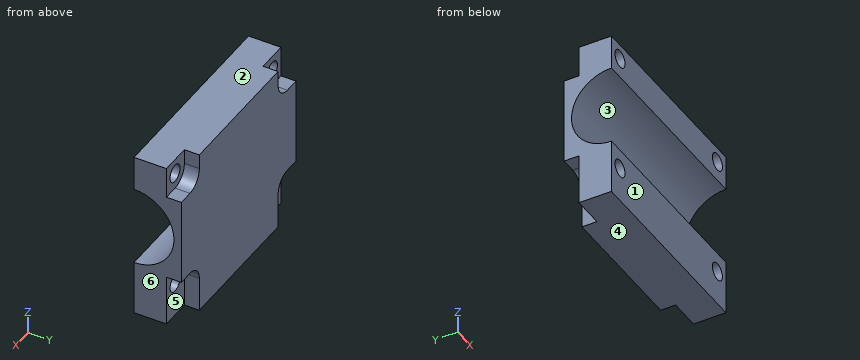
from build123d import *

# Parameters (mm, degrees)
SKETCH1_W            = 40
SKETCH1_H            = 34
SKETCH1_R            = 1.75
BOSS_EXTRUDE1_DEPTH  = 9.5
SKETCH2_R            = 8
CUT_EXTRUDE1_DEPTH   = 46.290727528
CUT_EXTRUDE2_DEPTH   = 3
MIRROR2_COPY_1_DEPTH = 3
SKETCH4_W            = 6.25
SKETCH4_H            = 4
CUT_EXTRUDE3_DEPTH   = 3


with BuildPart() as part:
    # Sketch1 → Boss-Extrude1 (new body)
    with BuildSketch(Plane(origin=(0, 0, 0), x_dir=(1, 0, 0), z_dir=(0, 1, 0))):
        with Locations((0, 2)):
            Rectangle(SKETCH1_W, SKETCH1_H)
        with Locations(Location((-17, 12, 0), (0, 0, 270))):
            Circle(SKETCH1_R, mode=Mode.SUBTRACT)
        with Locations(Location((17, 12, 0), (0, 0, 270))):
            Circle(SKETCH1_R, mode=Mode.SUBTRACT)
        with Locations(Location((17, -12, 0), (0, 0, 270))):
            Circle(SKETCH1_R, mode=Mode.SUBTRACT)
        with Locations(Location((-17, -12, 0), (0, 0, 270))):
            Circle(SKETCH1_R, mode=Mode.SUBTRACT)
    extrude(amount=BOSS_EXTRUDE1_DEPTH)

    # Sketch2 → Cut-Extrude1 (cut, through all)
    with BuildSketch(Plane(origin=(20, 0, 0), x_dir=(0, 0, -1), z_dir=(1, 0, 0))):
        Circle(SKETCH2_R)
    extrude(amount=-CUT_EXTRUDE1_DEPTH, mode=Mode.SUBTRACT)

    # Sketch3 → Cut-Extrude2 (cut)
    with BuildSketch(Plane(origin=(0, 9.5, 0), x_dir=(1, 0, 0), z_dir=(0, 1, 0))):
        with BuildLine():
            Line((-17, -8.75), (-20, -8.75))
            Line((-20, -8.75), (-20, -15))
            Line((-20, -15), (-13.75, -15))
            Line((-13.75, -15), (-13.75, -12))
            ThreePointArc((-13.75, -12), (-14.701902961, -9.701902961), (-17, -8.75))
        make_face()
    cut_extrude2 = extrude(amount=-CUT_EXTRUDE2_DEPTH, mode=Mode.SUBTRACT)

    # Mirror1: Cut-Extrude2 across plane
    add(cut_extrude2.mirror(Plane(origin=(0, 0, 0), x_dir=(0, 0, 1), z_dir=(1, 0, 0))), mode=Mode.SUBTRACT)

    # Mirror2: Cut-Extrude2 across plane
    add(cut_extrude2.mirror(Plane.XY), mode=Mode.SUBTRACT)

    # Mirror2 copy 1 sketch → Mirror2 copy 1 (cut)
    with BuildSketch(Plane(origin=(0, 9.5, 0), x_dir=(-1, 0, 0), z_dir=(0, 1, 0))):
        with BuildLine():
            Line((-17, -8.75), (-20, -8.75))
            Line((-20, -8.75), (-20, -15))
            Line((-20, -15), (-13.75, -15))
            Line((-13.75, -15), (-13.75, -12))
            ThreePointArc((-13.75, -12), (-14.701902961, -9.701902961), (-17, -8.75))
        make_face()
    extrude(amount=-MIRROR2_COPY_1_DEPTH, mode=Mode.SUBTRACT)

    # Sketch4 → Cut-Extrude3 (cut)
    with BuildSketch(Plane(origin=(0, 9.5, 0), x_dir=(1, 0, 0), z_dir=(0, 1, 0))):
        with Locations((-16.875, 17)):
            Rectangle(SKETCH4_W, SKETCH4_H)
        with Locations((16.875, 17)):
            Rectangle(SKETCH4_W, SKETCH4_H)
    extrude(amount=-CUT_EXTRUDE3_DEPTH, mode=Mode.SUBTRACT)


solid = part.part
The model under review builds one solid part; all positions refer to its coordinate system, in mm. Face numbers are marked on the shaded views. A direction names the side the tool comes from. Round coordinates to 2 decimals unless told otherwise and drop trailing zeros. Order: outer loops, then holes, each group sorted by start corner. A loop starts at its lowest first (then second) coordinate and runs counter-clockwise, first axis right, second up. Notation, with made-up numbers: (-6.5, 74.5) -> (32.5, 74.5) arc R21 ccw to (32.5, 93.5) -> close; hole circle Ø11 at (-34, 64.25). An arc over 180 degrees is marked (long way). Write item = value, one per line. Start each with the question number.
Item 1: For the marked faces 5 and 6, list the 3-axis set-ups (+Z, -Z, +X, -X, +Y, -Y) from which the entire face can be reached by the end or side of a thin tool; tool diameter is ignored.
Item 2: Consider section A-A on y = 1.5. Write out the cut boundary in (x, z), plus the area to 3 significant figures.
Item 3: Mouldability with a two-part tool opening along Z and no side actions: class the marked faces 1, 2, 3 and 4 as released by +Z, released by -Z, zero draft, split by the parting line, or undercut.
Item 4: Clearance check with flat-ended pins moving along their axes: pin 1 Ø5 at (x, y) = (16, 8.5) entering from +Z; pin 2 Ø2.5 at (y, z) = (8, 13.5) entering from +X; pin 3 Ø0.9 at (y, z) = (7.5, 14) entering from -X; pin 4 Ø3 at (x, z) = (-17, 12) entering from -Y. State where each tip first meets the part, or that it passes through.
Item 5: Consider section C-C on x = 0.5. Write out the cut boundary in (y, z).
Item 6: Consider section D-D on z = -9.5. Write out the cut boundary in (x, y).
Item 7: For line 1 along X through (y, z) = (4.25, -12); line 2 along Z through (x, y) = (17, 3.25); line 3 along Z through (x, y) = (17, 4.5), list the stretches that pass through material, from the lowest coordinate up.
Item 8: Consider section B-B on z = -16.5. Write out the cut boundary in (x, y), plus the area to 4 significant figures.
Conclusion:
q1.face_5 = -Z, +X, +Y
q1.face_6 = +Z, -Z, +X, +Y, -Y
q2.outline = (-20, -19) -> (20, -19) -> (20, -7.86) -> (-20, -7.86) -> close; (-20, 7.86) -> (20, 7.86) -> (20, 15) -> (-20, 15) -> close; hole circle Ø3.5 at (-17, -12); hole circle Ø3.5 at (-17, 12); hole circle Ø3.5 at (17, -12); hole circle Ø3.5 at (17, 12)
q2.area = 693 mm2
q3.face_1 = zero draft
q3.face_2 = released by +Z
q3.face_3 = undercut
q3.face_4 = released by -Z
q4.pin_1 = 15
q4.pin_2 = 13.75
q4.pin_3 = -13.75
q4.pin_4 = through
q5.outline = (0, -19) -> (9.5, -19) -> (9.5, 15) -> (0, 15) -> (0, 8) arc R8 cw to (0, -8) -> close
q6.outline = (-20, 0) -> (20, 0) -> (20, 6.5) -> (14.92, 6.5) -> (14.92, 9.5) -> (-14.92, 9.5) -> (-14.92, 6.5) -> (-20, 6.5) -> close
q7.line_1 = -20 to -18.75, -15.25 to 15.25, 18.75 to 20
q7.line_2 = -19 to -13.75, -10.25 to -7.31, 7.31 to 10.25, 13.75 to 15
q7.line_3 = -19 to -13.75, -10.25 to -6.61, 6.61 to 10.25, 13.75 to 15
q8.outline = (-20, 0) -> (20, 0) -> (20, 6.5) -> (13.75, 6.5) -> (13.75, 9.5) -> (-13.75, 9.5) -> (-13.75, 6.5) -> (-20, 6.5) -> close
q8.area = 342.5 mm2
